Work out the finished part from the listing and answer in its coordinate system (mm). A direction names the side the tool comes from. Coordinates: 2 decimals unless noted, no trailing zeros. Write each loop counter-clockwise with the first axis right and the second up, starting at its lowest first coordinate (ties: lowest second). Pieces come first, ordered by that corner, then holes. Notation, with made-up numbers: (-35.75, 80) - (-31.75, 80) arc R22 ccw to (-31.75, 100) - close; hole circle Ø5 at (-17.75, 32.5). An arc over 180 degrees is marked (long way). Answer as a JSON object with one key per item and string values. Group by question number.
from build123d import *

# Parameters (mm, degrees)
SCHIZZO1_W                   = 24.55
SCHIZZO1_H                   = 26.8
ESTRUSIONE_ESTRUSIONE1_DEPTH = 4
FORO_PER_VITE_M3_1_D         = 3.2
FORO_PER_VITE_M3_2_D         = 3.2
SCHIZZO5_R                   = 2
TAGLIO_ESTRUSIONE1_DEPTH     = 10
SCHIZZO6_W                   = 2
SCHIZZO6_H                   = 12
ESTRUSIONE_ESTRUSIONE2_DEPTH = 2
RACCORDO1_R                  = 1


with BuildPart() as part:
    # Schizzo1 → Estrusione-Estrusione1 (new body)
    with BuildSketch(Plane.XY):
        Rectangle(SCHIZZO1_W, SCHIZZO1_H)
    extrude(amount=ESTRUSIONE_ESTRUSIONE1_DEPTH)

    # Foro per Vite M3-1 (through all)
    with Locations(Plane.XY.offset(4)):
        with Locations((-4.205, 5), (4.295, 5), (4.295, -5), (-4.205, -5)):
            Hole(FORO_PER_VITE_M3_1_D / 2)

    # Foro per Vite M3-2 (through all)
    with Locations(Plane(origin=(-7.235, 10.5, 4), x_dir=(1, 0, 0), z_dir=(0, 0, 1))):
        with Locations((0, 0), (14.56, 0), (0, -21), (14.56, -21)):
            Hole(FORO_PER_VITE_M3_2_D / 2)

    # Schizzo5 → Taglio-Estrusione1 (cut)
    with BuildSketch(Plane.XY.offset(4)):
        with Locations((0.045, 0)):
            Circle(SCHIZZO5_R)
    extrude(amount=-TAGLIO_ESTRUSIONE1_DEPTH, mode=Mode.SUBTRACT)

    # Schizzo6 → Estrusione-Estrusione2 (add)
    with BuildSketch(Plane.XY.offset(4)):
        with Locations((-11.275, 0)):
            Rectangle(SCHIZZO6_W, SCHIZZO6_H)
    extrude(amount=ESTRUSIONE_ESTRUSIONE2_DEPTH)

    # Raccordo1
    raccordo1_edges = [part.edges().sort_by_distance(p)[0] for p in [
        (12.275, -13.4, 2),
        (-12.275, -13.4, 2),
        (-12.275, 13.4, 2),
        (12.275, 13.4, 2),
    ]]
    fillet(raccordo1_edges, radius=RACCORDO1_R)


solid = part.part
Q1. Section A-A on y = -5 is taken. Determine the outline of the cut face in (x, z) (3 decimals).
Q2. Flat-ended cylindrical pins translate along their axes: pin 1 Ø12 at (x, y) = (-4, -4) entering from +Z; pin 2 Ø1.6 at (y, z) = (2, 5.5) entering from +X (3 decimals); pin 3 Ø1.6 at (x, z) = (-11.5, 5) entering from -Y. Find the tip coordinate at first contact, or state that the pin passes through.
Q3. Section B-B on z = 1.8 is taken. Count the separate pieces of the cut face and the enclosed holes in it, plus the area to 3 significant figures.
Q4. Section C-C on y = 0 is taken. Determine the outline of the cut face in (x, z) (3 decimals).
Q5. A tool of negligible diameter and unlimited length cuts with its end or side. For faces 1 (the face through (-11, 6, 5)), 2 (the face through (-11, -6, 5)), 3 (the face through (-12.275, 0, 2)), from which of +Z, -Z, +X, -X, +Y, -Y can it reach the whole face along a straight path? Write none if from no direction.
Q6. Consider L1, parallel to Y at x = -3, z = 2.4; L2, parallel to X at y = -11.75, z = 3 (3 decimals); L3, parallel to Y at x = -2.75, z = 2.4. Determine where each line is inside the solid, lowest interval first. Write a range as from..to.
Q7. Section D-D on x = 3.25 is taken. Determine the outline of the cut face in (y, z), plus the area to 3 significant figures.
Q8. For a pull along X with two mould halves and no side action, classify faces 4 (the face through (-10.275, 0, 5)), 5 (the face through (3.56, 3.58, 1.97)), 6 (the face through (0, -2, 2)), 7 (the face through (-11.99, 13.1, 2.03)) as +X half, -X half, draft (parallel to the pull), parting line (faces both ways), or undercut.
Numbers:
{
 "1": {"outline": "(-12.275, 0) - (-5.805, 0) - (-5.805, 4) - (-10.275, 4) - (-10.275, 6) - (-12.275, 6) - close; (-2.605, 0) - (2.695, 0) - (2.695, 4) - (-2.605, 4) - close; (5.895, 0) - (12.275, 0) - (12.275, 4) - (5.895, 4) - close"},
 "2": {"pin 1": "stops at z = 4", "pin 2": "stops at x = -10.275", "pin 3": "stops at y = -6"},
 "3": {"separate pieces": "1", "enclosed holes": "9", "area": "580 mm²"},
 "4": {"outline": "(-12.275, 0) - (-1.955, 0) - (-1.955, 4) - (-10.275, 4) - (-10.275, 6) - (-12.275, 6) - close; (2.045, 0) - (12.275, 0) - (12.275, 4) - (2.045, 4) - close"},
 "5": {"face 1": "+Z, +X, -X, +Y", "face 2": "+Z, +X, -X, -Y", "face 3": "+Z, -Z, -X, +Y, -Y"},
 "6": {"L1": "y = -13.4..-6.05, -3.95..3.95, 6.05..13.4", "L2": "x = -12.275..-8.234, -6.236..6.326, 8.324..12.275", "L3": "y = -13.4..-5.67, -4.33..4.33, 5.67..13.4"},
 "7": {"outline": "(-13.4, 0) - (-6.21, 0) - (-6.21, 4) - (-13.4, 4) - close; (-3.79, 0) - (3.79, 0) - (3.79, 4) - (-3.79, 4) - close; (6.21, 0) - (13.4, 0) - (13.4, 4) - (6.21, 4) - close", "area": "87.8 mm²"},
 "8": {"face 4": "+X half", "face 5": "undercut", "face 6": "undercut", "face 7": "-X half"}
}
